Check sheet for the modelled part. Datum: model origin and axes. Units: mm. Face numbers are marked on the shaded views. A direction names the side the tool comes from. Give positions to 0.01 mm unless a question says otherwise; leave off trailing zeros. Write each loop counter-clockwise with the first axis right and the second up, starting at its lowest first coordinate (ties: lowest second). Pieces come first, ordered by that corner, then holes.
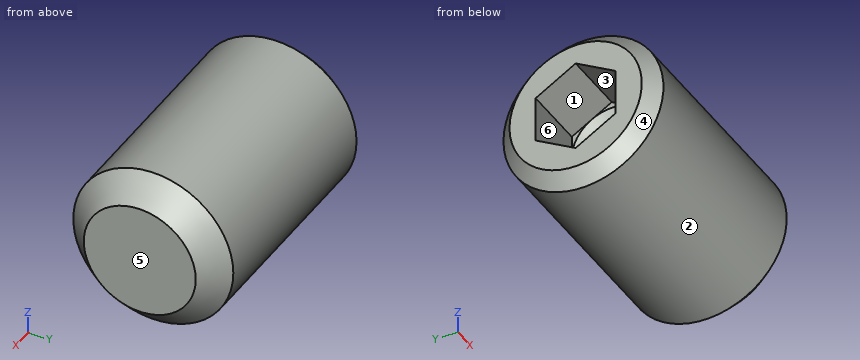
from build123d import *

# Parameters (mm, degrees)
HEXAGONSOCKET_DEPTH = 2


with BuildPart() as part:
    # Sketch1 → Base (revolve)
    with BuildSketch(Plane.XY):
        Polygon((0, 0), (8, 0), (8, 1.75), (7.25, 2.5), (0.433, 2.5), (0, 2.067), align=None)
    revolve(axis=Axis((-10.745014543, 0, 0), (1, 0, 0)))

    # Sketch2 → HexagonSocket (cut)
    with BuildSketch(Plane(origin=(0, -0.021932325, 0.010138848), x_dir=(0, 0, 1), z_dir=(-1, 0, 0))):
        Polygon((1.433236825, 0.021932325), (0.711548988, 1.271932325), (-0.731826685, 1.271932325), (-1.453514521, 0.021932325), (-0.731826685, -1.228067675), (0.711548988, -1.228067675), align=None)
    extrude(amount=-HEXAGONSOCKET_DEPTH, mode=Mode.SUBTRACT)

    # Sketch3 → Cut-Revolve1 (revolve, cut)
    with BuildSketch(Plane.XY):
        Polygon((2, 1.25), (2.721687837, 0), (2, 0), align=None)
    revolve(axis=Axis((-3.144113667, 0, 0), (1, 0, 0)), mode=Mode.SUBTRACT)


solid = part.part
1) Draft check along Z on the marked faces 3, 4, 5 and 6. Enter one of: +Z half, -Z half, draft (parallel to the pull), parting line (faces both ways), or undercut.
2) Sectioned sample at A-A on x = 4.5. Record the boundary of the cut face in (y, z).
3) Scan lines: L1, parallel to Y at x = 1, z = -0.1; L2, parallel to Z at x = 0.5, y = -0.7; L3, parallel to Y at x = 1.5, z = 0.55. Record each from-to range of solid material in increasing order.
4) Access from +Z, -Z, +X, -X, +Y, -Y to the whole of each face (thin tool, end or side, straight path). Record for the marked faces 1 and 2.
Answers below:
1. face 3: undercut
1. face 4: parting line
1. face 5: draft
1. face 6: undercut
2. outline: circle Ø5 at (0, 0)
3. L1: y = -2.5 to -1.25, 1.25 to 2.5
3. L2: z = -2.4 to -1.04, 1.04 to 2.4
3. L3: y = -2.44 to -1.25, 1.25 to 2.44
4. face 1: -X
4. face 2: +X, -X
